from build123d import *

# Parameters (mm, degrees)
F1_DEPTH = 19.05
F2_W     = 19.05
F2_H     = 7.62
F3_DEPTH = 88.901


with BuildPart() as f1:
    # F0 (on Top) → F1 (new body)
    with BuildSketch(Plane.XY):
        Polygon((44.45, -203.2), (44.45, 203.2), (10.735303, 203.2), (25.4, 177.8), (-25.4, 177.8), (-10.735303, 203.2), (-44.45, 203.2), (-44.45, -203.2), (-10.735303, -203.2), (-25.4, -177.8), (25.4, -177.8), (10.735303, -203.2), align=None)
    extrude(amount=F1_DEPTH)

    # F2 (on face) → F3 (cut, through all)
    with BuildSketch(Plane.YZ.offset(44.45)):
        with Locations((-174.625, 3.81)):
            Rectangle(F2_W, F2_H)
        with Locations((174.625, 3.81)):
            Rectangle(F2_W, F2_H)
    extrude(amount=-F3_DEPTH, mode=Mode.SUBTRACT)


solid = f1.part
Verification items for the finished model (mm, model axes). A direction names the side the tool comes from. Round coordinates to 2 decimals unless told otherwise and drop trailing zeros. Loops run counter-clockwise (first coordinate to the right, second up) from the corner with the lowest first, then second, coordinate; pieces in that order, holes last. Notation, with made-up numbers: (-10, -4.5) - (42, -4.5) arc R27 ccw to (42, 34.5) - close; hole circle Ø6 at (-16.75, 73.5). An arc over 180 degrees is marked (long way). Use one line per item in the form item = value.
1. Scan lines: probe 1 along Y at (x, z) = (-26, 4.25); probe 2 along Y at (x, z) = (-16, 11.5); probe 3 along Y at (x, z) = (5.5, 3). Record each from-to range of solid material in increasing order.
A:
probe_1 = -203.2 to -184.15, -165.1 to 165.1, 184.15 to 203.2
probe_2 = -203.2 to -194.08, -177.8 to 177.8, 194.08 to 203.2
probe_3 = -165.1 to 165.1
2. Section check D-D on x = -4. Record the cut outline in (y, z), and give its area (3 significant figures).
A:
outline = (-177.8, 7.62) - (-165.1, 7.62) - (-165.1, 0) - (165.1, 0) - (165.1, 7.62) - (177.8, 7.62) - (177.8, 19.05) - (-177.8, 19.05) - close
area = 6,580 mm²
3. Draft check along Y on faces 1 (the flat face through (-27, 203.2, 9)), 2 (the flat face through (-32, 194, 0)), 3 (the flat face through (17.965, 190.678, 9.392)). Enter one of: pulls with the +Y half, pulls with the -Y half, needs draft (parallel to the pull), parting line crosses it, or undercut.
A:
face_1 = pulls with the +Y half
face_2 = needs draft
face_3 = undercut
4. Section check B-B on x = 29. Record the cut outline in (y, z), and give its area (3 significant figures).
A:
outline = (-203.2, 0) - (-184.15, 0) - (-184.15, 7.62) - (-165.1, 7.62) - (-165.1, 0) - (165.1, 0) - (165.1, 7.62) - (184.15, 7.62) - (184.15, 0) - (203.2, 0) - (203.2, 19.05) - (-203.2, 19.05) - close
area = 7,450 mm²
5. Section check C-C on y = -173. Record the cut outline in (x, z), and give its area (3 significant figures).
A:
outline = (-44.45, 7.62) - (44.45, 7.62) - (44.45, 19.05) - (-44.45, 19.05) - close
area = 1,020 mm²
6. Gauge pin test, flat end, axial feed: pin 1 Ø1.5 at (x, z) = (-3, 15) entering from -Y. Record the tip position at first contact, or that the pin passes through.
A:
pin_1 = -177.8
7. Access from +Z, -Z, +X, -X, +Y, -Y to the whole of each face (thin tool, end or side, straight path). Record for faces 4 (the flat face through (44.45, -3, 9)), 5 (the flat face through (0, -177.8, 13)), 6 (the flat face through (33, 184.15, 4)).
A:
face_4 = +Z, -Z, +X, +Y, -Y
face_5 = +Z, -Z
face_6 = -Z, +X, -X
8. Section check A-A on z = 4.5. Record the cut outline in (x, y).
A:
outline = (-44.45, -203.2) - (-10.74, -203.2) - (-21.73, -184.15) - (-44.45, -184.15) - close; (-44.45, -165.1) - (44.45, -165.1) - (44.45, 165.1) - (-44.45, 165.1) - close; (-44.45, 184.15) - (-21.73, 184.15) - (-10.74, 203.2) - (-44.45, 203.2) - close; (10.74, -203.2) - (44.45, -203.2) - (44.45, -184.15) - (21.73, -184.15) - close; (10.74, 203.2) - (21.73, 184.15) - (44.45, 184.15) - (44.45, 203.2) - close
